For this review, take the finished solid that the model builds, in its own axes (mm). Coordinates: 2 decimals unless noted, no trailing zeros. Loops run counter-clockwise (first coordinate to the right, second up) from the corner with the lowest first, then second, coordinate; pieces in that order, holes last. Notation, with made-up numbers: (-6, 64.5) - (21, 64.5) arc R18 cw to (21, 79.5) - close; hole circle Ø2 at (-20, -14.5). An arc over 180 degrees is marked (long way). Answer as a JSON object with one key per item and string values. Group by question number.
Item 1: We need section A-A (x = 0). Give the boundary of the cut face in (y, z) (3 decimals), then the cut area to 3 significant figures.
Item 2: Clearance check with flat-ended pins moving along their axes: pin 1 (0.6 mm diameter, centred on y = 0, z = -4.5, fed in from +X); pin 2 (3 mm diameter, centred on x = 1.5, y = 5.5, fed in from -Z); pin 3 (0.6 mm diameter, centred on x = 1, y = -0.5, fed in from +Z); pin 4 (2.5 mm diameter, centred on x = 0, z = 0, fed in from +Y) (3 decimals). State where each tip first meets the part, or that it passes through.
Item 3: We need section D-D (z = 0.5). Give the boundary of the cut face in (x, y).
Item 4: We need section B-B (z = -1). Give the boundary of the cut face in (x, y).
Item 5: To check wall thickness, follow line 1 (Z direction, x = 0, y = -0.6) (3 decimals); line 2 (Y direction, x = -0.75, z = -4); line 3 (Z direction, x = 0.1, y = 6.25). State the ranges of each line that lie inside material, in increasing order.
Item 6: Mouldability with a two-part tool opening along X and no side actions: class faces 1 (the cylindrical face through (-0.434, -0.394, -1.952)), 2 (the flat face through (-0.2, 0, -2.4)) as released by +X, released by -X, zero draft, split by the parting line, or undercut.
Item 7: We need section C-C (x = -0.7). Give the boundary of the cut face in (y, z), then the cut area to 3 significant figures.
from build123d import *

# Parameters (mm, degrees)
F0_R     = 2
F1_DEPTH = 0.8
F2_R     = 0.4
F3_DEPTH = 10


with BuildPart() as f1:
    # F0 (on Front) → F1 (new body)
    with BuildSketch(Plane.XZ):
        with BuildLine():
            ThreePointArc((0.57, -2.879119), (2.267948, -1.862965), (2.935, 0))
            ThreePointArc((2.935, 0), (-1.862965, 2.267948), (-0.57, -2.879119))
            ThreePointArc((-0.57, -2.879119), (-0.286366, -2.920996), (0, -2.935))
            ThreePointArc((0, -2.935), (0.286366, -2.920996), (0.57, -2.879119))
        make_face()
        Circle(F0_R, mode=Mode.SUBTRACT)
        Polygon((1.5, -3.739119), (0.57, -3.739119), (0, -3.739119), (0, -5.855), (0.57, -5.855), (0.57, -4.879119), (1.5, -4.879119), align=None)
        with BuildLine():
            Line((0.57, -3.739119), (0.57, -2.879119))
            ThreePointArc((0.57, -2.879119), (0.286366, -2.920996), (0, -2.935))
            Line((0, -2.935), (0, -3.739119))
            Line((0, -3.739119), (0.57, -3.739119))
        make_face()
        with BuildLine():
            ThreePointArc((0, -2.935), (-0.286366, -2.920996), (-0.57, -2.879119))
            Line((-0.57, -2.879119), (-0.57, -3.739119))
            Line((-0.57, -3.739119), (0, -3.739119))
            Line((0, -3.739119), (0, -2.935))
        make_face()
        Polygon((0, -3.739119), (-0.57, -3.739119), (-1.5, -3.739119), (-1.5, -4.879119), (-0.57, -4.879119), (-0.57, -5.855), (0, -5.855), align=None)
    extrude(amount=F1_DEPTH)

    # F2 (on face) → F3 (join)
    with BuildSketch(Plane(origin=(0, 0, 0), x_dir=(-1, 0, 0), z_dir=(0, 1, 0))):
        with Locations((0, 2.469715)):
            Circle(F2_R)
    extrude(amount=F3_DEPTH)


solid = f1.part
Check sheet entries:
{
 "1": {"outline": "(-0.8, -5.855) - (0, -5.855) - (0, -2) - (-0.8, -2) - close; (-0.8, 2) - (0, 2) - (0, 2.07) - (10, 2.07) - (10, 2.87) - (0, 2.87) - (0, 2.935) - (-0.8, 2.935) - close", "area": "11.8 mm2"},
 "2": {"pin 1": "stops at x = 1.5", "pin 2": "stops at z = 2.07", "pin 3": "stops at z = 2.85", "pin 4": "passes through"},
 "3": {"outline": "(-2.89, -0.8) - (-1.94, -0.8) - (-1.94, 0) - (-2.89, 0) - close; (1.94, -0.8) - (2.89, -0.8) - (2.89, 0) - (1.94, 0) - close"},
 "4": {"outline": "(-2.76, -0.8) - (-1.73, -0.8) - (-1.73, 0) - (-2.76, 0) - close; (1.73, -0.8) - (2.76, -0.8) - (2.76, 0) - (1.73, 0) - close"},
 "5": {"line 1": "z = -5.855 to -2, 2 to 2.935", "line 2": "y = -0.8 to 0", "line 3": "z = 2.08 to 2.86"},
 "6": {"face 1": "undercut", "face 2": "zero draft"},
 "7": {"outline": "(-0.8, -4.88) - (0, -4.88) - (0, -3.74) - (-0.8, -3.74) - close; (-0.8, -2.85) - (0, -2.85) - (0, -1.87) - (-0.8, -1.87) - close; (-0.8, 1.87) - (0, 1.87) - (0, 2.85) - (-0.8, 2.85) - close", "area": "2.47 mm2"}
}
